```python
from build123d import *

# Parameters (mm, degrees)
F0_W     = 76.2
F0_H     = 88.9
F0_W_2   = 0.508
F0_W_3   = 75.184
F0_W_4   = 152.4
F1_DEPTH = 5.08


with BuildPart() as f1:
    # F0 (on Front) → F1 (new body)
    with BuildSketch(Plane.XZ):
        with Locations((-71.919513, -23.507463)):
            Rectangle(F0_W, F0_H)
        with Locations((-33.565513, -23.507463)):
            Rectangle(F0_W_2, F0_H)
        with Locations((4.280487, -23.507463)):
            Rectangle(F0_W_3, F0_H)
        with Locations((42.126487, -23.507463)):
            Rectangle(F0_W_2, F0_H)
        with Locations((118.580487, -23.507463)):
            Rectangle(F0_W_4, F0_H)
    extrude(amount=-F1_DEPTH)

    # F0 (on Front) → F2 (revolve)
    with BuildSketch(Plane.XZ):
        with Locations((-33.565513, -23.507463)):
            Rectangle(F0_W_2, F0_H)
    revolve(axis=Axis((-33.819513, 0, -23.507463), (0, 0, -1)))

    # F0 (on Front) → F3 (revolve)
    with BuildSketch(Plane.XZ):
        with Locations((42.126487, -23.507463)):
            Rectangle(F0_W_2, F0_H)
    revolve(axis=Axis((41.872487, 0, -23.507463), (0, 0, -1)))


solid = f1.part
```
Verification items for the finished model (mm, model axes). A direction names the side the tool comes from. Round coordinates to 2 decimals unless told otherwise and drop trailing zeros. Write each loop counter-clockwise with the first axis right and the second up, starting at its lowest first coordinate (ties: lowest second). Pieces come first, ordered by that corner, then holes. Notation, with made-up numbers: (-15.75, 59.25) -> (-0.75, 59.25) arc R19 cw to (-0.75, 93.25) -> close; hole circle Ø3 at (77.5, 21). An arc over 180 degrees is marked (long way). Write each question's results on one line, items separated by ' | '.
Q1. Sectioned sample at A-A, the plane z = 4.5. Record the boundary of the cut face in (x, y).
Derived:
outline: (-110.02, 0) -> (-34.33, 0) arc R0.51 ccw to (-33.31, 0) -> (41.36, 0) arc R0.51 ccw to (42.38, 0) -> (194.78, 0) -> (194.78, 5.08) -> (-110.02, 5.08) -> close
Q2. Go/stop test with a flat-tipped pin: pin 1 Ø12 at (x, z) = (23, -17) entering from -Y. Record where the tip stops, or that it passes through.
Derived:
pin 1: stops at y = 0
Q3. Sectioned sample at B-B, the plane x = 117. Record the boundary of the cut face in (y, z), and give its area (3 significant figures).
Derived:
outline: (0, -67.96) -> (5.08, -67.96) -> (5.08, 20.94) -> (0, 20.94) -> close | area: 452 mm²
Q4. Access from +Z, -Z, +X, -X, +Y, -Y to the whole of each face (thin tool, end or side, straight path). Record for faces 5 (the face through (45, 3, 20.943)), 6 (the face through (118, 0, -23)).
Derived:
face 5: +Z, +X, -X, +Y, -Y | face 6: +Z, -Z, +X, -Y
Q5. Thickness scan on probe 1 along X at (y, z) = (-0.15, -64); probe 2 along Y at (x, z) = (60.5, -23.5). Record the ranges inside material, lowest first.
Derived:
probe 1: x = -34.3 to -33.33, 41.39 to 42.36 | probe 2: y = 0 to 5.08
Q6. Draft check along X on faces 1 (the face through (194.78, 3, -24)), 2 (the face through (4, 0, -23)), 3 (the face through (-110.02, 3, -24)), 4 (the face through (-73, 0, -23)). Enter one of: released by +X, released by -X, zero draft, split by the parting line, or undercut.
Derived:
face 1: released by +X | face 2: undercut | face 3: released by -X | face 4: zero draft
